```python
from build123d import *

# Parameters (mm, degrees)
SKETCH1_W                = 80.3
SKETCH1_H                = 92.3
BOSS_EXTRUDE1_DEPTH      = 7.1
SKETCH2_W                = 65.8
SKETCH2_H                = 65.8
BOSS_EXTRUDE2_DEPTH      = 31.8
SKETCH3_R                = 9.6
BOSS_EXTRUDE3_DEPTH      = 52.1
CUT_EXTRUDE1_DEPTH       = 2.8
M5_CLEARANCE_SLOT1_D     = 5.5
FILLET1_R                = 4.8
M5_CLEARANCE_SLOT2_DEPTH = 7.1
SKETCH9_R                = 13.35
CUT_EXTRUDE2_DEPTH       = 1.8
SKETCH10_R               = 6.8
BOSS_EXTRUDE4_DEPTH      = 30
SKETCH11_R               = 15.6
BOSS_EXTRUDE5_DEPTH      = 49
FILLET2_R                = 15
CHAMFER1_SIZE            = 7.5
CHAMFER1_SIZE2           = 33.3


# Read off the part's stored shape, not the designer's step: M5 Clearance Slot2
with BuildPart() as part:
    # Sketch1 → Boss-Extrude1 (new body)
    with BuildSketch(Plane(origin=(0, 0, 0), x_dir=(1, 0, 0), z_dir=(0, 1, 0))):
        Rectangle(SKETCH1_W, SKETCH1_H)
    extrude(amount=BOSS_EXTRUDE1_DEPTH)

    # Sketch2 → Boss-Extrude2 (add)
    with BuildSketch(Plane.XZ):
        Rectangle(SKETCH2_W, SKETCH2_H)
    extrude(amount=BOSS_EXTRUDE2_DEPTH)

    # Sketch3 → Boss-Extrude3 (add)
    with BuildSketch(Plane.XZ.offset(31.8)):
        with Locations(Location((0, 0, 0), (0, 0, 90))):
            Circle(SKETCH3_R)
    extrude(amount=BOSS_EXTRUDE3_DEPTH)

    # Sketch4 → Cut-Extrude1 (cut)
    with BuildSketch(Plane(origin=(0, 7.1, 0), x_dir=(1, 0, 0), z_dir=(0, 1, 0))):
        with BuildLine():
            Line((-38.4, 33.1), (-38.4, -33.1))
            Line((-38.4, -33.1), (-20.9, -33.1))
            ThreePointArc((-20.9, -33.1), (-17.364466094, -34.564466094), (-15.9, -38.1))
            Line((-15.9, -38.1), (-15.9, -44.6))
            Line((-15.9, -44.6), (15.9, -44.6))
            Line((15.9, -44.6), (15.9, -38.1))
            ThreePointArc((15.9, -38.1), (17.364466094, -34.564466094), (20.9, -33.1))
            Line((20.9, -33.1), (38.4, -33.1))
            Line((38.4, -33.1), (38.4, 33.1))
            Line((38.4, 33.1), (20.9, 33.1))
            ThreePointArc((20.9, 33.1), (17.364466094, 34.564466094), (15.9, 38.1))
            Line((15.9, 38.1), (15.9, 44.6))
            Line((15.9, 44.6), (-15.9, 44.6))
            Line((-15.9, 44.6), (-15.9, 38.1))
            ThreePointArc((-15.9, 38.1), (-17.364466094, 34.564466094), (-20.9, 33.1))
            Line((-20.9, 33.1), (-38.4, 33.1))
        make_face()
    extrude(amount=-CUT_EXTRUDE1_DEPTH, mode=Mode.SUBTRACT)

    # M5 Clearance Slot1 (through all)
    with Locations(Plane(origin=(0, 7.1, 0), x_dir=(1, 0, 0), z_dir=(0, 1, 0))):
        with Locations((-33.45, 39.15), (33.45, 39.15), (33.45, -39.15), (-33.45, -39.15)):
            Hole(M5_CLEARANCE_SLOT1_D / 2)

    # Fillet1
    fillet1_edges = [part.edges().sort_by_distance(p)[0] for p in [
        (40.15, 3.55, 46.15),
        (-40.15, 3.55, 46.15),
        (-40.15, 3.55, -46.15),
        (40.15, 3.55, -46.15),
    ]]
    fillet(fillet1_edges, radius=FILLET1_R)

    # M5 Clearance Slot2 outline → M5 Clearance Slot2 (cut)
    with BuildSketch(Plane(origin=(0, 0, 0), x_dir=(1, 0, 0), z_dir=(0, 1, 0))):
        with BuildLine():
            Line((23.1, 35.9), (25.2, 35.9))
            ThreePointArc((25.2, 35.9), (28.95, 39.65), (25.2, 43.4))
            Line((25.2, 43.4), (23.1, 43.4))
            ThreePointArc((23.1, 43.4), (19.35, 39.65), (23.1, 35.9))
        make_face()
        with BuildLine():
            ThreePointArc((-23.1, 35.9), (-19.35, 39.65), (-23.1, 43.4))
            Line((-23.1, 43.4), (-25.2, 43.4))
            ThreePointArc((-25.2, 43.4), (-28.95, 39.65), (-25.2, 35.9))
            Line((-25.2, 35.9), (-23.1, 35.9))
        make_face()
        with BuildLine():
            Line((23.1, -43.4), (25.2, -43.4))
            ThreePointArc((25.2, -43.4), (28.95, -39.65), (25.2, -35.9))
            Line((25.2, -35.9), (23.1, -35.9))
            ThreePointArc((23.1, -35.9), (19.35, -39.65), (23.1, -43.4))
        make_face()
        with BuildLine():
            ThreePointArc((-23.1, -43.4), (-19.35, -39.65), (-23.1, -35.9))
            Line((-23.1, -35.9), (-25.2, -35.9))
            ThreePointArc((-25.2, -35.9), (-28.95, -39.65), (-25.2, -43.4))
            Line((-25.2, -43.4), (-23.1, -43.4))
        make_face()
    extrude(amount=M5_CLEARANCE_SLOT2_DEPTH, mode=Mode.SUBTRACT)

    # Sketch9 → Cut-Extrude2 (cut)
    with BuildSketch(Plane(origin=(0, 4.3, 0), x_dir=(1, 0, 0), z_dir=(0, 1, 0))):
        with Locations(Location((0, 0, 0), (0, 0, 270))):
            Circle(SKETCH9_R)
    extrude(amount=-CUT_EXTRUDE2_DEPTH, mode=Mode.SUBTRACT)

    # Sketch10 → Boss-Extrude4 (add)
    with BuildSketch(Plane(origin=(0, 2.5, 0), x_dir=(1, 0, 0), z_dir=(0, 1, 0))):
        with Locations(Location((0, 0, 0), (0, 0, 270))):
            Circle(SKETCH10_R)
    extrude(amount=BOSS_EXTRUDE4_DEPTH)

    # Sketch11 → Boss-Extrude5 (add)
    with BuildSketch(Plane(origin=(0, 32.5, 0), x_dir=(1, 0, 0), z_dir=(0, 1, 0))):
        with Locations(Location((0, 0, 0), (0, 0, 270))):
            Circle(SKETCH11_R)
    extrude(amount=BOSS_EXTRUDE5_DEPTH)

    # Fillet2
    fillet2_edges = [part.edges().sort_by_distance(p)[0] for p in [
        (0, 81.5, -15.6),
    ]]
    fillet(fillet2_edges, radius=FILLET2_R)

    # Chamfer1
    chamfer1_edges = [part.edges().sort_by_distance(p)[0] for p in [
        (0, 32.5, -15.6),
    ]]
    chamfer1_side = [part.faces().sort_by_distance(p)[0] for p in [
        (0, 32.5, -15.158765369),
    ]]
    chamfer(chamfer1_edges, length=CHAMFER1_SIZE, length2=CHAMFER1_SIZE2, reference=chamfer1_side[0])


solid = part.part
```
Verification items for the finished model (mm, model axes). A direction names the side the tool comes from. Round coordinates to 2 decimals unless told otherwise and drop trailing zeros. Write each loop counter-clockwise with the first axis right and the second up, starting at its lowest first coordinate (ties: lowest second). Pieces come first, ordered by that corner, then holes.
1. Gauge pin test, flat ends, axial feed: P1, Ø4, axis at y = -11, z = -29.5, coming from the -X side; P2, Ø23, axis at x = 13.5, z = 19.5, coming from the +Y side; P3, Ø3, axis at y = 5.5, z = 42.5, coming from the +X side; P4, Ø4, axis at y = 30, z = -1, coming from the +X side. Record the tip position at first contact, or that the pin passes through.
2. Scan lines: L1, parallel to X at y = 3.5, z = 39.15; L2, parallel to Z at x = -33, y = 5; L3, parallel to X at y = 2.95, z = 0. Record each from-to range of solid material in increasing order.
3. Access from +Z, -Z, +X, -X, +Y, -Y to the whole of each face (thin tool, end or side, straight path). Record for faces 5 (the cylindrical face through (-9.49, 66.15, -12.38)), 6 (the cylindrical face through (-28.95, 3.5, -39.73)), 7 (the cylindrical face through (38.71, 3.6, 44.78)), 8 (the flat face through (7, 32.5, -2)), 9 (the flat face through (-8, -31.8, 8)).
4. Draft check along X on faces 1 (the flat face through (0, -83.9, 0)), 2 (the conical face through (3.32, 45.68, 10.56)), 3 (the cylindrical face through (17.4, 5.72, -34.53)), 4 (the cylindrical face through (-19.35, 3.5, 39.73)). Enter one of: +X half, -X half, draft (parallel to the pull), parting line (faces both ways), or undercut.
5. Section check B-B on y = 11. Enter the section's corners in (x, z), plus the area to 3 significant figures.
6. Section check A-A on z = -29.5. Enter the section's corners in (x, y), plus the area to 3 significant figures.
7. Section check C-C on y = -57. Enter the section's corners in (x, z), plus the area to 3 significant figures.
Answer:
1. P1: stops at x = -32.9
1. P2: stops at y = 75.99
1. P3: stops at x = 40.15
1. P4: stops at x = 6.8
2. L1: x = -40.15 to -36.2, -30.7 to -28.92, -19.38 to 19.38, 28.92 to 30.7, 36.2 to 40.15
2. L2: z = -46.15 to -41.86, -36.44 to -33.1, 33.1 to 36.44, 41.86 to 46.15
2. L3: x = -40.15 to -13.35, -6.8 to 6.8, 13.35 to 40.15
3. face 5: +Y
3. face 6: +Y, -Y
3. face 7: +Z, +X, +Y, -Y
3. face 8: none
3. face 9: -Y
4. face 1: draft
4. face 2: parting line
4. face 3: undercut
4. face 4: undercut
5. outline: circle Ø13.6 at (0, 0)
5. area: 145 mm2
6. outline: (-40.15, 0) - (-32.9, 0) - (-32.9, -31.8) - (32.9, -31.8) - (32.9, 0) - (40.15, 0) - (40.15, 7.1) - (38.4, 7.1) - (38.4, 4.3) - (-38.4, 4.3) - (-38.4, 7.1) - (-40.15, 7.1) - close
6. area: 2,450 mm2
7. outline: circle Ø19.2 at (0, 0)
7. area: 290 mm2
